Autodesk Fusion 360 part; units mm, degrees
sketch "Skizze1" plane through (0, 0, 0) normal (0, 1, 0) x (1, 0, 0)
  line L0 (0, 0) -> (164, 0)
  line L1 (164, 0) -> (164, -18)
  line L2 (164, -18) -> (0, -18)
  line L3 (0, -18) -> (0, 0)
  dimension "d1" = 18
  dimension "d2" = 164
extrude "Extrusion1" add sketch "Skizze1" along normal blind 8
fillet "Abrundung1" radius 5 4 edges at (0, 4, 18) (164, 4, 18) (0, 4, 0) (164, 4, 0)
sketch "Skizze2" plane through (0, 0, 0) normal (0, 1, 0) x (1, 0, 0)
  line L0 (-8, -19.5) -> (172, -19.5)
  line L1 (172, -19.5) -> (172, 0.5)
  line L2 (172, 0.5) -> (-8, 0.5)
  line L3 (-8, 0.5) -> (-8, -19.5)
  line L4 (-8, -9) -> (172, -9) construction
  circle A0 centre (-3, -9) radius 1.75
  circle A1 centre (167, -9) radius 1.75
  point P0 (0, -13)
  point P1 (164, -13)
  dimension "d7" = 0.5
  dimension "d8" = 19.5
  dimension "d9" = 9
  dimension "d10" = 3
  dimension "d11" = 3
  dimension "d12" = 3.5
  dimension "d13" = 5
  dimension "d14" = 5
extrude "Extrusion2" add sketch "Skizze2" against normal blind 1
fillet "Abrundung2" radius 6 4 edges at (172, -0.5, 19.5) (172, -0.5, -0.5) (-8, -0.5, 19.5) (-8, -0.5, -0.5)
extrude "Extrusion3" cut 1 faces at (56.3333, 8, 12) along direction (0, -1, 0) blind 6
sketch "Skizze3" plane through (0, 2, 0) normal (0, 1, 0) x (-1, 0, 0)
  arc A0 (-164, 5) -> (-159, 0) centre (-159, 5) ccw
  line L0 (-159, 0) -> (-5, 0)
  arc A1 (-5, 0) -> (0, 5) centre (-5, 5) ccw
  line L1 (0, 5) -> (0, 13)
  arc A2 (0, 13) -> (-5, 18) centre (-5, 13) ccw
  line L2 (-5, 18) -> (-159, 18)
  arc A3 (-159, 18) -> (-164, 13) centre (-159, 13) ccw
  line L3 (-164, 13) -> (-164, 5)
  line L4 (-96, 14.5) -> (-84, 14.5)
  line L5 (-84, 14.5) -> (-84, 3)
  line L6 (-84, 3) -> (-96, 3)
  line L7 (-96, 3) -> (-96, 14.5)
  dimension "d21" = 68
  dimension "d22" = 3
  dimension "d23" = 3.5
  dimension "d24" = 12
extrude "Extrusion4" add sketch "Skizze3" along normal blind 3 contours L4 L5 L6 L7
sketch "Skizze4" plane through (0, 2, 0) normal (0, 1, 0) x (-1, 0, 0)
  line L0 (-96, 3) -> (-96, 14.5)
  line L1 (-96, 14.5) -> (-84, 14.5)
  line L2 (-84, 14.5) -> (-84, 3)
  line L3 (-84, 3) -> (-96, 3)
  arc A0 (-164, 5) -> (-159, 0) centre (-159, 5) ccw
  line L4 (-159, 0) -> (-5, 0)
  arc A1 (-5, 0) -> (0, 5) centre (-5, 5) ccw
  line L5 (0, 5) -> (0, 13)
  arc A2 (0, 13) -> (-5, 18) centre (-5, 13) ccw
  line L6 (-5, 18) -> (-159, 18)
  arc A3 (-159, 18) -> (-164, 13) centre (-159, 13) ccw
  line L7 (-164, 13) -> (-164, 5)
  line L8 (-99, 18) -> (-81, 18)
  line L9 (-81, 18) -> (-81, 0)
  line L10 (-81, 0) -> (-99, 0)
  line L11 (-99, 0) -> (-99, 18)
  dimension "d27" = 3.5
  dimension "d28" = 3
  dimension "d29" = 3
  dimension "d30" = 3
extrude "Extrusion5" add sketch "Skizze4" along normal blind 5 contours L4 L6 L8 L9 L10 L11
sketch "Skizze5" plane through (0, 5, 0) normal (0, 1, 0) x (-1, 0, 0)
  line L0 (-96, 3) -> (-84, 3)
  line L1 (-84, 3) -> (-84, 14.5)
  line L2 (-84, 14.5) -> (-96, 14.5)
  line L3 (-96, 14.5) -> (-96, 3)
  line L4 (-95.5, 14) -> (-84.5, 14)
  line L5 (-84.5, 14) -> (-84.5, 3.5)
  line L6 (-84.5, 3.5) -> (-95.5, 3.5)
  line L7 (-95.5, 3.5) -> (-95.5, 14)
  dimension "d33" = 0.5
  dimension "d34" = 0.5
  dimension "d35" = 0.5
  dimension "d36" = 0.5
extrude "Extrusion6" cut sketch "Skizze5" against normal blind 13 contours L4 L5 L6 L7
sketch "Skizze6" plane through (0, -1, 0) normal (0, -1, 0) x (1, 0, 0)
  line L0 (84.5, 3.5) -> (84.5, 14)
  line L1 (84.5, 14) -> (95.5, 14)
  line L2 (95.5, 14) -> (95.5, 3.5)
  line L3 (95.5, 3.5) -> (84.5, 3.5)
  arc A0 (-8, 5.5) -> (-2, -0.5) centre (-2, 5.5) ccw
  line L4 (-2, -0.5) -> (166, -0.5)
  arc A1 (166, -0.5) -> (172, 5.5) centre (166, 5.5) ccw
  line L5 (172, 5.5) -> (172, 13.5)
  arc A2 (172, 13.5) -> (166, 19.5) centre (166, 13.5) ccw
  line L6 (166, 19.5) -> (-2, 19.5)
  arc A3 (-2, 19.5) -> (-8, 13.5) centre (-2, 13.5) ccw
  line L7 (-8, 13.5) -> (-8, 5.5)
  circle A4 centre (-3, 9) radius 1.75
  circle A5 centre (167, 9) radius 1.75
  line L8 (84, 14.5) -> (96, 14.5)
  line L9 (96, 14.5) -> (96, 3)
  line L10 (96, 3) -> (84, 3)
  line L11 (84, 3) -> (84, 14.5)
  dimension "d39" = 0.5
  dimension "d40" = 0.5
  dimension "d41" = 0.5
  dimension "d42" = 0.5
extrude "Extrusion7" cut sketch "Skizze6" against normal blind 5 contours L8 L9 L10 L11
chamfer "Fase1" distance 5 angle 45 2 edges at (99, 2, 9) (81, 2, 9)
Can you work these out from the model? Positions are in its coordinate system, mm. A direction names the side the tool comes from. Round coordinates to 2 decimals unless told otherwise and drop trailing zeros. Loops run counter-clockwise (first coordinate to the right, second up) from the corner with the lowest first, then second, coordinate; pieces in that order, holes last. Notation, with made-up numbers: (-12.5, -20.5) - (35.5, -20.5) arc R24 cw to (35.5, 9.5) - close; hole circle Ø5 at (33, 49.5). An arc over 180 degrees is marked (long way). Answer in a Markdown table with one row per item. Add a question column.
Q1. Which directions (+Z, -Z, +X, -X, +Y, -Y) give clear straight access to the entire face, cutting with the end or side of a thin tool? Please do faces 1 (the cylindrical face through (162, 1, 17)), 2 (the flat face through (90, 1, 14.5)), 3 (the cylindrical face through (163, 1, 2)), 4 (the flat face through (90.5, 5, 3.2)), 5 (the flat face through (81, 2, 18)).
Q2. I want a section at A-A on z = 9. Count the separate pieces of the cut face and the enclosed holes in it, and give its area (3 significant figures).
Q3. We'd pull the mould along X, two halves only. Please class faces 6 (the cylindrical face through (170.196, -0.507, 1.211)), 7 (the flat face through (89.5, 4, 3.2)), 8 (the cylindrical face through (2, 1, 1)), 9 (the cylindrical face through (168.669, -0.493, 8.474)): pulls with the +X half, pulls with the -X half, needs draft (parallel to the pull), parting line crosses it, or undercut.
Q4. I need wall thicknesses on L1, parallel to X at y = -0.75, z = 9; L2, parallel to X at y = -0.5, z = 12; L3, parallel to Y at x = 75.5, z = 15.25. Which ranges of each line are inside material? Lowest first, please.
Q5. I want a section at B-B on x = 128. List the corners of the cut face in (y, z) for me, and give its area (3 significant figures).
Q6. For pin 1 Ø1.5 at (y, z) = (1, 9) entering from +X; pin 2 Ø2.5 at (x, y) = (89.5, 0.5) entering from +Z; pin 3 Ø4 at (y, z) = (1.5, 16.5) entering from -X; pin 4 Ø3 at (x, z) = (-3, 9) entering from +Y, each with a flat end and sliding along its axis, tell me the tip position at first contact or that it passes through.
A:
| question | item | result |
|---|---|---|
| 1 | face 1 | +Z, +X, +Y |
| 1 | face 2 | -Y |
| 1 | face 3 | -Z, +X, +Y |
| 1 | face 4 | +Y |
| 1 | face 5 | +Z, +X, -X, +Y |
| 2 | separate pieces | 4 |
| 2 | enclosed holes | 0 |
| 2 | area | 521 mm^2 |
| 3 | face 6 | pulls with the +X half |
| 3 | face 7 | undercut |
| 3 | face 8 | pulls with the -X half |
| 3 | face 9 | undercut |
| 4 | L1 | -8 to -4.75, -1.25 to 84, 96 to 165.25, 168.75 to 172 |
| 4 | L2 | -8 to 84, 96 to 172 |
| 4 | L3 | -1 to 2 |
| 5 | outline | (-1, -0.5) - (0, -0.5) - (0, 0) - (2, 0) - (2, 18) - (0, 18) - (0, 19.5) - (-1, 19.5) - close |
| 5 | area | 56.0 mm^2 |
| 6 | pin 1 | x = 164 |
| 6 | pin 2 | z = 19.5 |
| 6 | pin 3 | x = -7.76 |
| 6 | pin 4 | through |
